from build123d import *

# Parameters (mm, degrees)
F2_SIZE = 1.27
F3_SIZE = 1.27


with BuildPart() as f1:
    # F0 (on Front) → F1 (revolve)
    with BuildSketch(Plane.XZ):
        Polygon((-30, 0), (0, 0), (0, 4.293243), (-26, 4.293243), (-26, 8.360523), (-20, 13), (-30, 13), align=None)
    revolve(axis=Axis((0, 0, 2.146621), (0, 0, -1)))

    # F2
    f2_edges = [f1.edges().sort_by_distance(p)[0] for p in [
        (30, 0, 13),
    ]]
    chamfer(f2_edges, length=F2_SIZE)

    # F3
    f3_edges = [f1.edges().sort_by_distance(p)[0] for p in [
        (30, 0, 0),
    ]]
    chamfer(f3_edges, length=F3_SIZE)


solid = f1.part
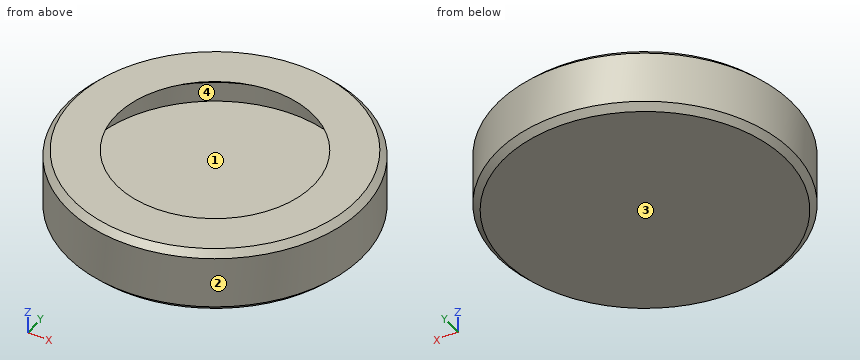
Work out the finished part from the listing and answer in its coordinate system (mm). Face numbers are marked on the shaded views. Round coordinates to 2 decimals unless told otherwise and drop trailing zeros. Loops run counter-clockwise (first coordinate to the right, second up) from the corner with the lowest first, then second, coordinate; pieces in that order, holes last. Notation, with made-up numbers: M 84.25,12 L 115.25,12 A19 cw 115.25,41 Z; hole C 34,-37.5 d2. An arc over 180 degrees is marked long. One line per question, with ' | ' between items. Start each with the question number.
(1) A cutting plane is placed at C-C on z = 7. Write down the section's boundary in (x, y), plus the area to 3 significant figures.
(2) Flat-ended cylindrical pins translate along their axes: pin 1 Ø2 at (x, y) = (-3.5, -2.5) entering from -Z; pin 2 Ø10 at (x, y) = (5.5, -6.5) entering from +Z; pin 3 Ø1 at (x, z) = (-22.5, 5) entering from +Y; pin 4 Ø4 at (y, z) = (-10.5, 5) entering from -X. Find the tip coordinate at first contact, or state that the pin passes through.
(3) For a pull along X with two mould halves and no side action, classify the marked faces 1, 2, 3 and 4 as released by +X, released by -X, zero draft, split by the parting line, or undercut.
(4) A cutting plane is placed at A-A on y = 0. Write down the section's boundary in (x, z), plus the area to 3 significant figures.
(5) Find the intervals of material crossed by line 1 (Y direction, x = 0, z = 6.95); line 2 (Y direction, x = -12, z = 4.5); line 3 (Z direction, x = -6.5, y = 10), in increasing order.
Geometry check:
1) outline: C 0,0 d60; hole C 0,0 d52 | area: 704 mm²
2) pin 1: stops at z = 0 | pin 2: stops at z = 4.29 | pin 3: stops at y = 20.4 | pin 4: stops at x = -28.77
3) face 1: undercut | face 2: split by the parting line | face 3: zero draft | face 4: undercut
4) outline: M -30,1.27 L -28.73,0 L 28.73,0 L 30,1.27 L 30,11.73 L 28.73,13 L 20,13 L 26,8.36 L 26,4.29 L -26,4.29 L -26,8.36 L -20,13 L -28.73,13 L -30,11.73 Z | area: 352 mm²
5) line 1: y = -30 to -26, 26 to 30 | line 2: y = -27.5 to -23.07, 23.07 to 27.5 | line 3: z = 0 to 4.29
